The listing builds one solid part. Answer for the finished solid, in the listing's coordinates (mm). Give positions to 0.01 mm unless a question says otherwise; leave off trailing zeros. Write each loop counter-clockwise with the first axis right and the second up, starting at its lowest first coordinate (ties: lowest second). Pieces come first, ordered by that corner, then holes. Notation, with made-up numbers: (-22, -0.5) -> (33, -0.5) arc R14 ccw to (33, 4.5) -> close; hole circle Ø5 at (-33.75, 34). An arc over 180 degrees is marked (long way). Put each result on its own line as item: value. Start each with the question number.
1) A cutting plane is placed at D-D (z = -0.65). Write down the section's boundary in (x, y).
2) A cutting plane is placed at C-C (x = 1.25). Write down the section's boundary in (y, z).
3) Flat-ended cylindrical pins translate along their axes: pin 1 Ø0.5 at (x, y) = (1.5, 4) entering from -Z; pin 2 Ø0.7 at (y, z) = (4.5, -1.5) entering from -X; pin 3 Ø0.5 at (y, z) = (-1, -1.5) entering from +X. Find the tip coordinate at first contact, or state that the pin passes through.
4) A cutting plane is placed at B-B (x = 1.95). Write down the section's boundary in (y, z).
5) For a pull along X with two mould halves and no side action, classify faces 1 (the flat face through (2.54, 1, -1)), 2 (the flat face through (0, 2.54, -1)), 3 (the flat face through (1, 1, 0)) as released by +X, released by -X, zero draft, split by the parting line, or undercut.
6) Find the intervals of material crossed by line 1 along X through (y, z) = (5.5, -1.2); line 2 along Y through (x, z) = (0.65, -0.1); line 3 along Y through (x, z) = (-0.3, -1.15), in increasing order. Write a range as from..to.
7) A cutting plane is placed at A-A (y = 5.5). Write down the section's boundary in (x, z), then the cut area to 3 significant figures.
from build123d import *
from OCP.BRepFilletAPI import BRepFilletAPI_MakeChamfer

# Parameters (mm, degrees)
SKETCH1_W                     = 2.54
SKETCH1_H                     = 2.54
MAIN_BODY_DEPTH               = 2.54
SKETCH3_W                     = 1.778
SKETCH3_H                     = 0.381
CUT_EXTRUDE1_DEPTH            = 5.399409051
CUT_EXTRUDE2_DEPTH            = 5.399409051
BODY_PATTERN_COUNT            = 2
BODY_PATTERN_PITCH            = 2.54
PIN_START                     = -5.54
SKETCH2_W                     = 0.64
SKETCH2_H                     = 0.64
PIN_DEPTH                     = 11.54
CHAMFER1_SIZE                 = 0.508
CHAMFER1_SIZE2                = 0.1905
CHAMFER2_SIZE                 = 0.1905
CHAMFER2_SIZE2                = 0.508
PIN_PATTERN_COUNT             = 2
PIN_PATTERN_PITCH             = 2.54
CHAMFER1_OF_PIN_PATTERN_SIZE  = 0.508
CHAMFER1_OF_PIN_PATTERN_SIZE2 = 0.1905
CHAMFER2_OF_PIN_PATTERN_SIZE2 = 0.1905
CHAMFER2_OF_PIN_PATTERN_SIZE  = 0.508


with BuildPart() as part:
    # Sketch1 → Main Body (new body)
    with BuildSketch(Plane(origin=(0, 0, 0), x_dir=(1, 0, 0), z_dir=(0, 1, 0))):
        with Locations((1.27, 1.27)):
            Rectangle(SKETCH1_W, SKETCH1_H)
    main_body = extrude(amount=MAIN_BODY_DEPTH)

    # Sketch3 → Cut-Extrude1 (cut, through all)
    with BuildSketch(Plane.ZY):
        with Locations((-1.27, 0.1905)):
            Rectangle(SKETCH3_W, SKETCH3_H)
    cut_extrude1 = extrude(amount=-CUT_EXTRUDE1_DEPTH, mode=Mode.SUBTRACT)

    # Sketch4 → Cut-Extrude2 (cut, through all)
    with BuildSketch(Plane(origin=(0, 2.54, 0), x_dir=(1, 0, 0), z_dir=(0, 1, 0))):
        Polygon((0.254, 2.54), (0, 2.54), (0, 2.032), align=None)
        Polygon((2.54, 2.54), (2.286, 2.54), (2.54, 2.032), align=None)
        Polygon((0.254, 0), (0, 0.508), (0, 0), align=None)
        Polygon((2.54, 0), (2.286, 0), (2.54, 0.508), align=None)
    cut_extrude2 = extrude(amount=-CUT_EXTRUDE2_DEPTH, mode=Mode.SUBTRACT)

    # Body Pattern: Main Body, Cut-Extrude1, Cut-Extrude2 ×2
    with Locations(*[(-i * BODY_PATTERN_PITCH, 0, 0) for i in range(1, BODY_PATTERN_COUNT)]):
        add(main_body)
        add(cut_extrude1, mode=Mode.SUBTRACT)
        add(cut_extrude2, mode=Mode.SUBTRACT)

    # Sketch2 → Pin (add)
    with BuildSketch(Plane(origin=(0, 2.54, 0), x_dir=(1, 0, 0), z_dir=(0, 1, 0)).offset(PIN_START)):
        with Locations((1.27, 1.27)):
            Rectangle(SKETCH2_W, SKETCH2_H)
    pin = extrude(amount=PIN_DEPTH)

    # Chamfer1: one chamfer whose edges measure the first distance from different faces: ONE call of the kernel's chamfer builder (chamfer() names one face for all edges)
    chamfer1_edges_1 = [part.edges().sort_by_distance(p)[0] for p in [
        (0.95, 8.54, -1.27),
    ]]
    chamfer1_side_1 = [part.faces().sort_by_distance(p)[0] for p in [
        (0.95, 5.54, -1.27),
    ]]
    chamfer1_edges_2 = [part.edges().sort_by_distance(p)[0] for p in [
        (1.27, 8.54, -0.95),
    ]]
    chamfer1_side_2 = [part.faces().sort_by_distance(p)[0] for p in [
        (1.27, 5.54, -0.95),
    ]]
    chamfer1_edges_3 = [part.edges().sort_by_distance(p)[0] for p in [
        (1.59, 8.54, -1.27),
    ]]
    chamfer1_side_3 = [part.faces().sort_by_distance(p)[0] for p in [
        (1.59, 5.54, -1.27),
    ]]
    chamfer1_edges_4 = [part.edges().sort_by_distance(p)[0] for p in [
        (1.27, 8.54, -1.59),
    ]]
    chamfer1_side_4 = [part.faces().sort_by_distance(p)[0] for p in [
        (1.27, 5.54, -1.59),
    ]]
    chamfer1 = BRepFilletAPI_MakeChamfer(part.part.solid().wrapped)
    for e in chamfer1_edges_1:
        chamfer1.Add(CHAMFER1_SIZE, CHAMFER1_SIZE2, e.wrapped, chamfer1_side_1[0].wrapped)  # the first distance lies on this face
    for e in chamfer1_edges_2:
        chamfer1.Add(CHAMFER1_SIZE, CHAMFER1_SIZE2, e.wrapped, chamfer1_side_2[0].wrapped)  # the first distance lies on this face
    for e in chamfer1_edges_3:
        chamfer1.Add(CHAMFER1_SIZE, CHAMFER1_SIZE2, e.wrapped, chamfer1_side_3[0].wrapped)  # the first distance lies on this face
    for e in chamfer1_edges_4:
        chamfer1.Add(CHAMFER1_SIZE, CHAMFER1_SIZE2, e.wrapped, chamfer1_side_4[0].wrapped)  # the first distance lies on this face
    add(Compound.cast(chamfer1.Shape()), mode=Mode.REPLACE)

    # Chamfer2
    chamfer2_edges = [part.edges().sort_by_distance(p)[0] for p in [
        (1.27, -3, -0.95),
        (1.59, -3, -1.27),
        (1.27, -3, -1.59),
        (0.95, -3, -1.27),
    ]]
    chamfer2_side = [part.faces().sort_by_distance(p)[0] for p in [
        (1.27, -3, -1.27),
    ]]
    chamfer(chamfer2_edges, length=CHAMFER2_SIZE, length2=CHAMFER2_SIZE2, reference=chamfer2_side[0])

    # Pin Pattern: Pin ×2
    with Locations(*[(-i * PIN_PATTERN_PITCH, 0, 0) for i in range(1, PIN_PATTERN_COUNT)]):
        add(pin)

    # Chamfer1 of Pin Pattern: one chamfer whose edges measure the first distance from different faces: ONE call of the kernel's chamfer builder (chamfer() names one face for all edges)
    chamfer1_of_pin_pattern_edges_1 = [part.edges().sort_by_distance(p)[0] for p in [
        (-1.59, 8.54, -1.27),
    ]]
    chamfer1_of_pin_pattern_side_1 = [part.faces().sort_by_distance(p)[0] for p in [
        (-1.59, 5.54, -1.27),
    ]]
    chamfer1_of_pin_pattern_edges_2 = [part.edges().sort_by_distance(p)[0] for p in [
        (-1.27, 8.54, -0.95),
    ]]
    chamfer1_of_pin_pattern_side_2 = [part.faces().sort_by_distance(p)[0] for p in [
        (-1.27, 5.54, -0.95),
    ]]
    chamfer1_of_pin_pattern_edges_3 = [part.edges().sort_by_distance(p)[0] for p in [
        (-0.95, 8.54, -1.27),
    ]]
    chamfer1_of_pin_pattern_side_3 = [part.faces().sort_by_distance(p)[0] for p in [
        (-0.95, 5.54, -1.27),
    ]]
    chamfer1_of_pin_pattern_edges_4 = [part.edges().sort_by_distance(p)[0] for p in [
        (-1.27, 8.54, -1.59),
    ]]
    chamfer1_of_pin_pattern_side_4 = [part.faces().sort_by_distance(p)[0] for p in [
        (-1.27, 5.54, -1.59),
    ]]
    chamfer1_of_pin_pattern = BRepFilletAPI_MakeChamfer(part.part.solid().wrapped)
    for e in chamfer1_of_pin_pattern_edges_1:
        chamfer1_of_pin_pattern.Add(CHAMFER1_OF_PIN_PATTERN_SIZE, CHAMFER1_OF_PIN_PATTERN_SIZE2, e.wrapped, chamfer1_of_pin_pattern_side_1[0].wrapped)  # the first distance lies on this face
    for e in chamfer1_of_pin_pattern_edges_2:
        chamfer1_of_pin_pattern.Add(CHAMFER1_OF_PIN_PATTERN_SIZE, CHAMFER1_OF_PIN_PATTERN_SIZE2, e.wrapped, chamfer1_of_pin_pattern_side_2[0].wrapped)  # the first distance lies on this face
    for e in chamfer1_of_pin_pattern_edges_3:
        chamfer1_of_pin_pattern.Add(CHAMFER1_OF_PIN_PATTERN_SIZE, CHAMFER1_OF_PIN_PATTERN_SIZE2, e.wrapped, chamfer1_of_pin_pattern_side_3[0].wrapped)  # the first distance lies on this face
    for e in chamfer1_of_pin_pattern_edges_4:
        chamfer1_of_pin_pattern.Add(CHAMFER1_OF_PIN_PATTERN_SIZE, CHAMFER1_OF_PIN_PATTERN_SIZE2, e.wrapped, chamfer1_of_pin_pattern_side_4[0].wrapped)  # the first distance lies on this face
    add(Compound.cast(chamfer1_of_pin_pattern.Shape()), mode=Mode.REPLACE)

    # Chamfer2 of Pin Pattern
    chamfer2_of_pin_pattern_edges = [part.edges().sort_by_distance(p)[0] for p in [
        (-1.27, -3, -0.95),
        (-0.95, -3, -1.27),
        (-1.27, -3, -1.59),
        (-1.59, -3, -1.27),
    ]]
    chamfer(chamfer2_of_pin_pattern_edges, length=CHAMFER2_OF_PIN_PATTERN_SIZE, length2=CHAMFER2_OF_PIN_PATTERN_SIZE2)


solid = part.part
Reply:
1. outline: (-2.54, 0.38) -> (2.54, 0.38) -> (2.54, 2.54) -> (-2.54, 2.54) -> close
2. outline: (-3, -1.4) -> (-2.49, -1.59) -> (0.38, -1.59) -> (0.38, -2.16) -> (0, -2.16) -> (0, -2.54) -> (2.54, -2.54) -> (2.54, -1.59) -> (8.03, -1.59) -> (8.54, -1.4) -> (8.54, -1.14) -> (8.03, -0.95) -> (2.54, -0.95) -> (2.54, 0) -> (0, 0) -> (0, -0.38) -> (0.38, -0.38) -> (0.38, -0.95) -> (-2.49, -0.95) -> (-3, -1.14) -> close
3. pin 1: stops at z = -1.59
3. pin 2: stops at x = -1.59
3. pin 3: stops at x = 1.59
4. outline: (0, -2.54) -> (2.54, -2.54) -> (2.54, 0) -> (0, 0) -> (0, -0.38) -> (0.38, -0.38) -> (0.38, -2.16) -> (0, -2.16) -> close
5. face 1: released by +X
5. face 2: undercut
5. face 3: zero draft
6. line 1: x = -1.59..-0.95, 0.95..1.59
6. line 2: y = 0..2.54
6. line 3: y = 0.38..2.54
7. outline: (-1.59, -1.59) -> (-0.95, -1.59) -> (-0.95, -0.95) -> (-1.59, -0.95) -> close; (0.95, -1.59) -> (1.59, -1.59) -> (1.59, -0.95) -> (0.95, -0.95) -> close
7. area: 0.819 mm2
